Autodesk Inventor part; units mm, degrees
ref_plane "YZ Plane" through (0, 0, 0) normal (1, 0, 0) x (0, 1, 0)
ref_plane "XZ Plane" through (0, 0, 0) normal (0, 1, 0) x (-1, 0, 0)
ref_plane "XY Plane" through (0, 0, 0) normal (0, 0, 1) x (1, 0, 0)
sketch "Boceto1" plane through (0, 0, 0) normal (0, 0, 1) x (1, 0, 0)
  line L0 (0, 0) -> (40.5, 0)
  line L1 (40.5, 0) -> (40.5, 28)
  line L2 (40.5, 28) -> (0, 28)
  line L3 (0, 28) -> (0, 0)
extrude "Extrusión1" add sketch "Boceto1" against normal blind 20
sketch "Boceto2" plane through (0, 0, 0) normal (0, 0, 1) x (1, 0, 0)
  line L0 (0, 0) -> (0, 28)
  line L1 (0, 28) -> (-7, 28)
  line L2 (-7, 28) -> (-7, 30.5)
  line L3 (-7, 30.5) -> (47.5, 30.5)
  line L4 (47.5, 30.5) -> (47.5, 28)
  line L5 (40.5, 28) -> (40.5, 0)
  line L6 (47.5, 28) -> (40.5, 28)
  line L7 (40.5, 28) -> (0, 28)
extrude "Extrusión2" add sketch "Boceto2" against normal blind 20
sketch "Boceto3" plane through (0, 0, 0) normal (0, 0, 1) x (1, 0, 0)
  line L0 (0, 35.5) -> (0, 30.5)
  line L1 (47.5, 30.5) -> (-7, 30.5)
  line L2 (0, 30.5) -> (40.5, 30.5)
  line L3 (0, 35.5) -> (40.5, 35.5)
  line L4 (40.5, 35.5) -> (40.5, 30.5)
  point P0 (0, 0)
extrude "Extrusión3" add sketch "Boceto3" against normal blind 20
sketch "Boceto4" plane through (0, 35.5, 0) normal (0, 1, 0) x (1, 0, 0)
  circle A0 centre (45.5, 5.0013) radius 2
  circle A1 centre (45.5, 15.0013) radius 2
  line L0 (-7, 0) -> (-7, 20)
  circle A2 centre (-5, 15.0013) radius 2
  circle A3 centre (-5, 5.0013) radius 2
  point P0 (0, 0)
hole "Agujero1" at (-5, 35.5, -15.0013) at (-5, 35.5, -5.0013) at (45.5, 35.5, -5.0013) at (45.5, 35.5, -15.0013) direction (0, -1, 0) diameter 4 end through all
sketch "Boceto5" plane through (0, 35.5, 0) normal (0, 1, 0) x (1, 0, 0)
  arc A0 (24.3765, 2) -> (24.3765, 18) centre (29.5, 10) ccw
  arc A1 (6.1878, 13) -> (6.1878, 7) centre (6.1878, 10) ccw
  line L0 (6.1878, 13) -> (6.1878, 15)
  line L1 (6.1878, 7) -> (6.1878, 5)
  line L2 (0, 20) -> (40.5, 20)
  line L3 (6.1878, 15) -> (6.1878, 18)
  line L4 (6.1878, 5) -> (6.1878, 2)
  line L5 (6.1878, 2) -> (24.3765, 2)
  line L6 (6.1878, 18) -> (24.3765, 18)
  circle A2 centre (29.5, 10) radius 9.5
  point P0 (24.3765, 18)
  point P1 (24.3765, 2)
  point P2 (24.3765, 2)
  point P3 (24.3765, 18)
extrude "Extrusión4" add sketch "Boceto5" along normal blind 3 contours A2 A0
extrude "Extrusión5" add sketch "Boceto5" along normal blind 2 contours L5 L4 L1 A1 L0 L3 L6 A2
sketch "Boceto6" plane through (29.5, 38.5, -10) normal (0, 1, 0) x (1, 0, 0)
  circle A0 centre (0, 0) radius 3
  point P0 (-29.5, -10)
extrude "Extrusión6" add sketch "Boceto6" along normal blind 3
thread "Rosca1"
sketch "Boceto7" plane through (29.5, 41.5, -10) normal (0, 1, 0) x (1, 0, 0)
  point P0 (-29.5, -10)
properties part number "Servo" material "Oro"
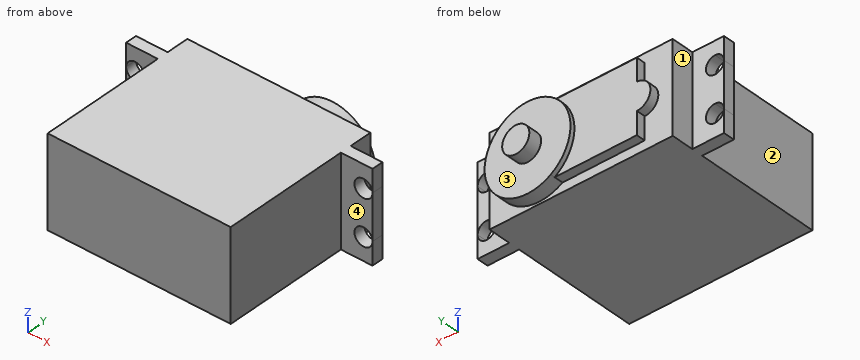
Source: CAD feature listing. Evaluate the final solid. Frame: model axes, mm. Face numbers are marked on the shaded views. A direction names the side the tool comes from. Give positions to 0.01 mm unless a question says otherwise; leave off trailing zeros. Order: outer loops, then holes, each group sorted by start corner. A loop starts at its lowest first (then second) coordinate and runs counter-clockwise, first axis right, second up. Notation, with made-up numbers: (58.5, 26.25) -> (98.5, 26.25) arc R16 cw to (98.5, 39.25) -> close; hole circle Ø9 at (-4.5, -2.75). An arc over 180 degrees is marked (long way). Write item = value, one per line.
Item 1: Section query C-C (y = 10.5). Output: boundary loops of the cut face in (x, z), then the cut area to 3 significant figures.
Check result:
outline = (0, -20) -> (40.5, -20) -> (40.5, 0) -> (0, 0) -> close
area = 810 mm²
Item 2: Contact query for flat-ended pins moving along their axis: pin 1 (8 mm diameter, centred on x = 10, z = -7, fed in from +Y); pin 2 (5.5 mm diameter, centred on y = 33.5, z = -6, fed in from +X); pin 3 (7.5 mm diameter, centred on x = 45, z = -6.5, fed in from -Y). Output: stop coordinate, or through.
Check result:
pin_1 = 37.5
pin_2 = 40.5
pin_3 = 28
Item 3: Section query D-D (x = 7.5). Output: boundary loops of the cut face in (y, z), then the cut area to 3 significant figures.
Check result:
outline = (0, -20) -> (35.5, -20) -> (35.5, -18) -> (37.5, -18) -> (37.5, -2) -> (35.5, -2) -> (35.5, 0) -> (0, 0) -> close
area = 742 mm²
Item 4: Ray query, probe 1 along Z at (x, y) = (45.5, 29.55); probe 2 along Y at (x, z) = (18, -15.5); probe 3 along X at (y, z) = (18, -13.25). Return the intervals inside material, ascending.
Check result:
probe_1 = -20 to -17, -13 to -7, -3 to 0
probe_2 = 0 to 37.5
probe_3 = 0 to 40.5
Item 5: Section query B-B (z = -7.75). Output: boundary loops of the cut face in (x, y), then the cut area to 3 significant figures.
Check result:
outline = (-7, 28) -> (0, 28) -> (0, 0) -> (40.5, 0) -> (40.5, 28) -> (47.5, 28) -> (47.5, 30.5) -> (40.5, 30.5) -> (40.5, 35.5) -> (38.73, 35.5) -> (38.73, 38.5) -> (31.48, 38.5) -> (31.48, 41.5) -> (27.52, 41.5) -> (27.52, 38.5) -> (20.27, 38.5) -> (20.27, 37.5) -> (4.2, 37.5) -> (4.2, 35.5) -> (0, 35.5) -> (0, 30.5) -> (-7, 30.5) -> close
area = 1,570 mm²
Item 6: Set-up query: the marked faces 1, 2, 3 and 4. Return all of +Z, -Z, +X, -X, +Y, -Y with unobstructed straight access to the full face (end or side cutting, diameter ignored); none if empty.
Check result:
face_1 = +Z, -Z, -X, +Y
face_2 = +Z, -Z, -X, -Y
face_3 = +Y
face_4 = +Z, -Z, +X, -Y
Item 7: Section query A-A (x = 29.5). Output: boundary loops of the cut face in (y, z).
Check result:
outline = (0, -20) -> (35.5, -20) -> (35.5, -19.5) -> (38.5, -19.5) -> (38.5, -13) -> (41.5, -13) -> (41.5, -7) -> (38.5, -7) -> (38.5, -0.5) -> (35.5, -0.5) -> (35.5, 0) -> (0, 0) -> close
